from build123d import *

# Parameters (mm, degrees)
BOSS_EXTRUDE1_DEPTH = 6.5
BOSS_EXTRUDE2_DEPTH = 6
CUT_EXTRUDE1_DEPTH  = 48.507894081
CHAMFER1_SIZE       = 3


with BuildPart() as part:
    # Sketch1 → Boss-Extrude1 (new body)
    with BuildSketch(Plane.XY):
        with BuildLine():
            Line((-5, -7.483314774), (-5, -22))
            Line((-5, -22), (5, -22))
            Line((5, -22), (5, -7.483314774))
            ThreePointArc((5, -7.483314774), (0, 9), (-5, -7.483314774))
        make_face()
        with BuildLine():
            Line((2.574956832, 3.99150314), (-4.147449153, 2.315419081))
            ThreePointArc((-4.147449153, 2.315419081), (-4.6089047, -1.149129004), (-2.574956832, -3.99150314))
            Line((-2.574956832, -3.99150314), (4.147449153, -2.315419081))
            ThreePointArc((4.147449153, -2.315419081), (4.6089047, 1.149129004), (2.574956832, 3.99150314))
        make_face(mode=Mode.SUBTRACT)
    extrude(amount=BOSS_EXTRUDE1_DEPTH)

    # Sketch2 → Boss-Extrude2 (add, symmetric)
    with BuildSketch(Plane(origin=(0, 0, 0), x_dir=(0, 0, -1), z_dir=(1, 0, 0))):
        with BuildLine():
            Line((-12, -20), (0, -20))
            Line((0, -20), (0, -40))
            Line((0, -40), (-3.75, -40))
            Line((-3.75, -40), (-3.75, -32))
            ThreePointArc((-3.75, -32), (-12, -23.75), (-20.25, -32))
            Line((-20.25, -32), (-20.25, -40))
            Line((-20.25, -40), (-24, -40))
            Line((-24, -40), (-24, -32))
            ThreePointArc((-24, -32), (-20.485281374, -23.514718626), (-12, -20))
        make_face()
    extrude(amount=BOSS_EXTRUDE2_DEPTH, both=True)

    # Sketch4 → Cut-Extrude1 (cut, through all)
    with BuildSketch(Plane.XY.offset(24)):
        with BuildLine():
            Line((-2.75, -32), (-2.75, -40))
            Line((-2.75, -40), (2.75, -40))
            Line((2.75, -40), (2.75, -32))
            ThreePointArc((2.75, -32), (0, -29.25), (-2.75, -32))
        make_face()
    extrude(amount=-CUT_EXTRUDE1_DEPTH, mode=Mode.SUBTRACT)

    # Chamfer1
    # the kernel refuses this chamfer: 3 mm, written as the material it adds along each edge
    with BuildSketch(Plane(origin=(-5, -20, 6.5), x_dir=(0.02749587661058619, 0.9996219169112968, 0), z_dir=(0, 0, -1))) as chamfer1_piece_1_section:
        Polygon((CHAMFER1_SIZE * 0.999621916911, -CHAMFER1_SIZE * 0.0274958766106), (-CHAMFER1_SIZE * 0.0274958766106, -CHAMFER1_SIZE * 0.999621916911), (0, 0), align=None)
    chamfer1_piece_1 = extrude(amount=6.5, mode=Mode.PRIVATE)
    chamfer1_piece_1 = split(chamfer1_piece_1, bisect_by=Plane(origin=(-6, -18.713879333, 3.25), z_dir=(1, 0, 0)), keep=Keep.TOP, mode=Mode.PRIVATE)
    add(chamfer1_piece_1)
    with BuildSketch(Plane(origin=(-5, -20, 6.5), x_dir=(0, -0.02749587661058678, 0.9996219169112968), z_dir=(1, 0, 0))) as chamfer1_piece_2:
        Polygon((CHAMFER1_SIZE * 0.999621916911, -CHAMFER1_SIZE * 0.0274958766106), (-CHAMFER1_SIZE * 0.0274958766106, -CHAMFER1_SIZE * 0.999621916911), (0, 0), align=None)
    extrude(amount=10)
    with BuildSketch(Plane(origin=(5, -20, 0), x_dir=(0.9996219169112968, -0.02749587661058678, 0), z_dir=(0, 0, 1))) as chamfer1_piece_3_section:
        Polygon((CHAMFER1_SIZE * 0.999621916911, CHAMFER1_SIZE * 0.0274958766106), (-CHAMFER1_SIZE * 0.0274958766106, CHAMFER1_SIZE * 0.999621916911), (0, 0), align=None)
    chamfer1_piece_3 = extrude(amount=6.5, mode=Mode.PRIVATE)
    chamfer1_piece_3 = split(chamfer1_piece_3, bisect_by=Plane(origin=(6, -18.713879333, 3.25), z_dir=(-1, 0, 0)), keep=Keep.TOP, mode=Mode.PRIVATE)
    add(chamfer1_piece_3)
    with BuildSketch(Plane(origin=(-5, -20, 14.215048964), x_dir=(0.02749587661058619, 0.9996219169112968, 0), z_dir=(0, 0, -1))) as chamfer1_piece_4a_section:
        Polygon((CHAMFER1_SIZE * 0.999621916911, -CHAMFER1_SIZE * 0.0274958766106), (-CHAMFER1_SIZE * 0.0274958766106, -CHAMFER1_SIZE * 0.999621916911), (0, 0), align=None)
    chamfer1_piece_4a = extrude(amount=14.215048964, mode=Mode.PRIVATE)
    chamfer1_piece_4a = split(chamfer1_piece_4a, bisect_by=Plane(origin=(-5.42545334, -18.713879333, 6.5), z_dir=(0, 0, 1)), keep=Keep.TOP, mode=Mode.PRIVATE)
    chamfer1_piece_4a = split(chamfer1_piece_4a, bisect_by=Plane(origin=(-6, -18.713879333, 10.357524482), z_dir=(1, 0, 0)), keep=Keep.TOP, mode=Mode.PRIVATE)
    with BuildSketch(Plane(origin=(-12.715048964, -20, 6.5), x_dir=(0, -0.02749587661058678, 0.9996219169112968), z_dir=(1, 0, 0))) as chamfer1_piece_4b_section:
        Polygon((CHAMFER1_SIZE * 0.999621916911, -CHAMFER1_SIZE * 0.0274958766106), (-CHAMFER1_SIZE * 0.0274958766106, -CHAMFER1_SIZE * 0.999621916911), (0, 0), align=None)
    chamfer1_piece_4b = extrude(amount=17.715048964, mode=Mode.PRIVATE)
    chamfer1_piece_4b = split(chamfer1_piece_4b, bisect_by=Plane(origin=(-5, -19.01061912, 7.48938088), z_dir=(-1, 0, 0)), keep=Keep.TOP, mode=Mode.PRIVATE)
    chamfer1_piece_4b = split(chamfer1_piece_4b, bisect_by=Plane(origin=(-6, -19.01061912, 7.48938088), z_dir=(1, 0, 0)), keep=Keep.TOP, mode=Mode.PRIVATE)
    chamfer1_piece_4 = chamfer1_piece_4a & chamfer1_piece_4b
    add(chamfer1_piece_4)
    with BuildSketch(Plane(origin=(5, -20, 0), x_dir=(0.9996219169112968, -0.02749587661058678, 0), z_dir=(0, 0, 1))) as chamfer1_piece_5a_section:
        Polygon((CHAMFER1_SIZE * 0.999621916911, CHAMFER1_SIZE * 0.0274958766106), (-CHAMFER1_SIZE * 0.0274958766106, CHAMFER1_SIZE * 0.999621916911), (0, 0), align=None)
    chamfer1_piece_5a = extrude(amount=14.215048964, mode=Mode.PRIVATE)
    chamfer1_piece_5a = split(chamfer1_piece_5a, bisect_by=Plane(origin=(6, -18.713879333, 10.357524482), z_dir=(-1, 0, 0)), keep=Keep.TOP, mode=Mode.PRIVATE)
    chamfer1_piece_5a = split(chamfer1_piece_5a, bisect_by=Plane(origin=(5.42545334, -18.713879333, 6.5), z_dir=(0, 0, 1)), keep=Keep.TOP, mode=Mode.PRIVATE)
    with BuildSketch(Plane(origin=(-5, -20, 6.5), x_dir=(0, -0.02749587661058678, 0.9996219169112968), z_dir=(1, 0, 0))) as chamfer1_piece_5b_section:
        Polygon((CHAMFER1_SIZE * 0.999621916911, -CHAMFER1_SIZE * 0.0274958766106), (-CHAMFER1_SIZE * 0.0274958766106, -CHAMFER1_SIZE * 0.999621916911), (0, 0), align=None)
    chamfer1_piece_5b = extrude(amount=17.715048964, mode=Mode.PRIVATE)
    chamfer1_piece_5b = split(chamfer1_piece_5b, bisect_by=Plane(origin=(6, -19.01061912, 7.48938088), z_dir=(-1, 0, 0)), keep=Keep.TOP, mode=Mode.PRIVATE)
    chamfer1_piece_5b = split(chamfer1_piece_5b, bisect_by=Plane(origin=(5, -19.01061912, 7.48938088), z_dir=(1, 0, 0)), keep=Keep.TOP, mode=Mode.PRIVATE)
    chamfer1_piece_5 = chamfer1_piece_5a & chamfer1_piece_5b
    add(chamfer1_piece_5)


solid = part.part
Check sheet for the modelled part. Datum: model origin and axes. Units: mm. A direction names the side the tool comes from. Coordinates: 2 decimals unless noted, no trailing zeros. Loops run counter-clockwise (first coordinate to the right, second up) from the corner with the lowest first, then second, coordinate; pieces in that order, holes last. Notation, with made-up numbers: (-19, 2.5) -> (28, 2.5) arc R14 cw to (28, 12.5) -> close; hole circle Ø3 at (20.25, -26). An arc over 180 degrees is marked (long way). Write item = value, one per line. Start each with the question number.
1. Tool access check on faces 4 (the flat face through (-2.75, -36, 2)), 5 (the flat face through (5, -12, 3)), 6 (the flat face through (6, -24, 7)), 7 (the flat face through (4, -36, 3.75)). Record the directions out of +Z, -Z, +X, -X, +Y, -Y that give a thin tool (end or side, any length) a straight path to the whole face; none if there is none.
2. Section check A-A on x = 1. Record the cut outline in (y, z), then the cut area to 3 significant figures.
3. Section check C-C on z = 5. Record the cut outline in (x, y).
4. Section check D-D on z = 21.75. Record the cut outline in (x, y).
5. Draft check along Y on faces 1 (the flat face through (-4, -40, 22)), 2 (the cylindrical face through (4.62, 1.1, 3.2)), 3 (the flat face through (0, -4, 6.5)). Enter one of: released by +Y, released by -Y, zero draft, split by the parting line, or undercut.
6. Material ranges on line 1 (X direction, y = -38, z = 20.75); line 2 (Z direction, x = 1.25, y = 4); line 3 (X direction, y = -20.5, z = 10), recorded low to high.
7. Section check B-B on y = -24.5. Record the cut outline in (x, z), then the cut area to 3 significant figures.
8. Depth check by flat-ended pin: P1, Ø8, axis at x = 0.5, z = 16, coming from the -Y side; P2, Ø3, axis at y = -14.5, z = 2.5, coming from the +X side; P3, Ø2, axis at y = -11, z = 2.5, coming from the -X side. Enter the tip coordinate at first touch or a pass-through.
Responses:
q1.face_4 = +Z, -Z, -Y
q1.face_5 = +Z, -Z, +X
q1.face_6 = +Z, -Z, +X, -Y
q1.face_7 = +X, -X, -Y
q2.outline = (-29.44, 0) -> (-3.1, 0) -> (-3.1, 6.5) -> (-17, 6.5) -> (-20, 9.5) -> (-20, 12) arc R12 ccw to (-29.44, 23.72) -> (-29.44, 19.84) arc R8.25 cw to (-29.44, 4.16) -> close; (3.6, 0) -> (8.94, 0) -> (8.94, 6.5) -> (3.6, 6.5) -> close
q2.area = 280 mm2
q3.outline = (-6, -27.63) -> (6, -27.63) -> (6, -18) -> (5, -17) -> (5, -7.48) arc R9 ccw (long way) to (-5, -7.48) -> (-5, -17) -> (-6, -18) -> close; hole (-4.15, 2.32) arc R4.75 ccw to (-2.57, -3.99) -> (4.15, -2.32) arc R4.75 ccw to (2.57, 3.99) -> close
q4.outline = (-6, -40) -> (-2.75, -40) -> (-2.75, -32) arc R2.75 cw to (2.75, -32) -> (2.75, -40) -> (6, -40) -> (6, -25) -> (-6, -25) -> close
q5.face_1 = released by -Y
q5.face_2 = undercut
q5.face_3 = zero draft
q6.line_1 = -6 to -2.75, 2.75 to 6
q6.line_2 = 0 to 6.5
q6.line_3 = -6 to 6
q7.outline = (-6, 0) -> (6, 0) -> (6, 8.56) -> (-6, 8.56) -> close; (-6, 15.44) -> (6, 15.44) -> (6, 21.37) -> (-6, 21.37) -> close
q7.area = 174 mm2
q8.P1 = -29.62
q8.P2 = 5
q8.P3 = -5
